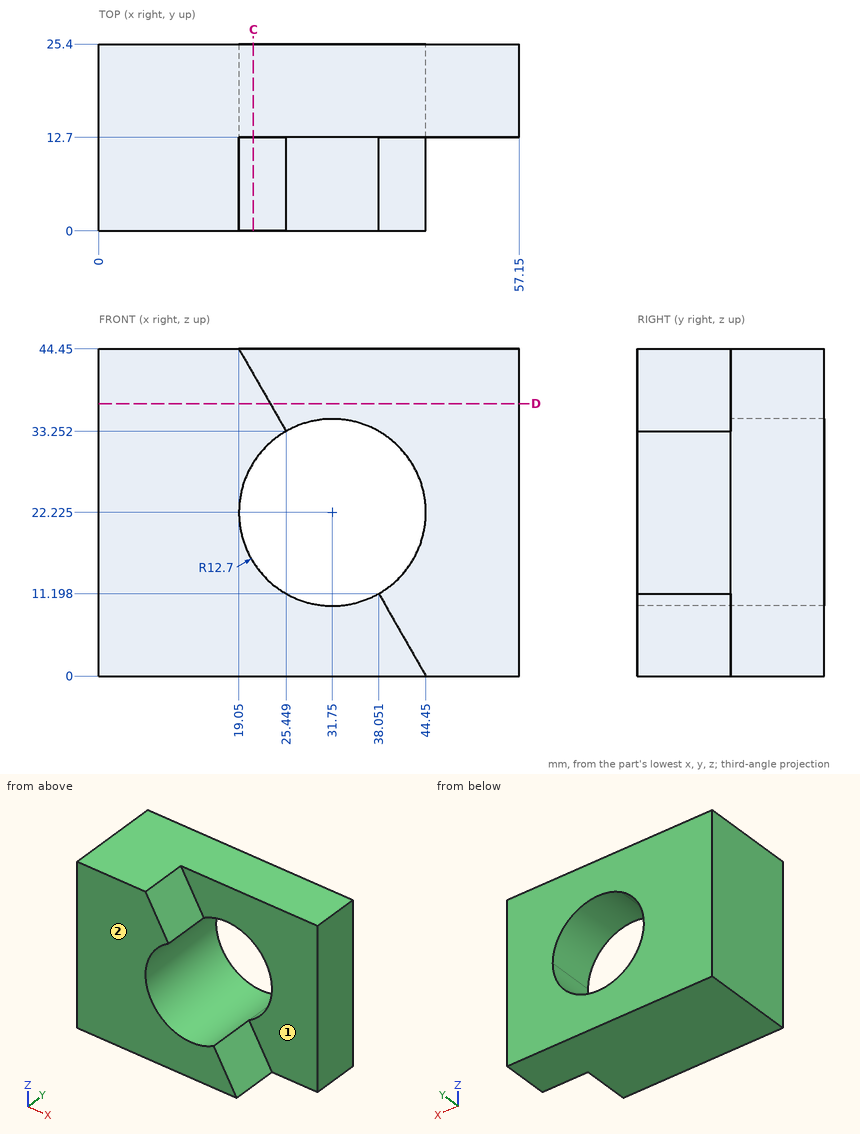
Can you work these out from the drawing? Everything is in mm from the part's minimum corner. A direction names the side the tool comes from. Give positions to 0.01 mm unless a question says otherwise; leave off trailing zeros. Order: outer loops, then holes, each group sorted by start corner. A loop starts at its lowest first (then second) coordinate and runs counter-clockwise, first axis right, second up. Notation, with made-up numbers: (53.25, 35.5) -> (107.25, 35.5) arc R23 cw to (107.25, 73.5) -> close; hole circle Ø6 at (47, -15). An arc over 180 degrees is marked (long way). Return JSON: item names as keys, results as strings.
1. For pin 1 Ø2 at (x, y) = (43.5, 10.5) entering from +Z; pin 2 Ø1 at (x, z) = (48.5, 11) entering from -Y; pin 3 Ø3 at (y, z) = (8, 9) entering from +X (1 decimal), each with a flat end and sliding along its axis, tell me the tip position at first contact or that it passes through.
Answer list:
{"pin 1": "stops at z = 3.41", "pin 2": "stops at y = 12.7", "pin 3": "stops at x = 40.2"}
2. I need wall thicknesses on line 1 (Z direction, x = 35, y = 22.25); line 2 (Y direction, x = 45.5, z = 27); line 3 (Z direction, x = 37.5, y = 18.5). Which ranges of each line are inside material? Lowest first, please. Write a range as from..to.
Answer list:
{"line 1": "z = 0..9.95, 34.5..44.45", "line 2": "y = 12.7..25.4", "line 3": "z = 0..10.9, 33.55..44.45"}
3. On a 3-axis mill with a long thin cutter (end or side, diameter ignored), from which of +Z, -Z, +X, -X, +Y, -Y can I reach the whole of each face in a straight line? I mean the marked faces 1 and 2. Say none if no direction works.
Answer list:
{"face 1": "+Z, +X, -Y", "face 2": "+Z, -Z, +X, -X, -Y"}
4. Imagine slicing it at D-D on z = 37. List the corners of the cut face in (x, y) for me, then the cut area to 3 significant figures.
Answer list:
{"outline": "(0, 0) -> (23.31, 0) -> (23.31, 12.7) -> (57.15, 12.7) -> (57.15, 25.4) -> (0, 25.4) -> close", "area": "1,020 mm2"}
5. Imagine slicing it at C-C on x = 21. List the corners of the cut face in (y, z) for me.
Answer list:
{"outline": "(0, 0) -> (25.4, 0) -> (25.4, 15.46) -> (0, 15.46) -> close; (0, 28.99) -> (25.4, 28.99) -> (25.4, 44.45) -> (12.7, 44.45) -> (12.7, 41.04) -> (0, 41.04) -> close"}
